```python
from build123d import *

# Parameters (mm, degrees)
SKETCH_1_W             = 43
SKETCH_1_H             = 39
BODY_DEPTH             = 1.5
SKETCH_3_R             = 1.3
OLED_PILLAR_DEPTH      = 5
OLED_WINDOW_REACH      = 31.745
SKETCH_2_W             = 34
SKETCH_2_H             = 18
SKETCH_4_W             = 43
SKETCH_4_H             = 39
SKETCH_4_W_2           = 40
SKETCH_4_H_2           = 36
FARMFEELWALL_DEPTH     = 20
MICRO5PIN_WINDOW_REACH = 53.276
SKETCH_7_W             = 12
SKETCH_7_H             = 5
RESET_WINDOW_REACH     = 50.819
SKETCH_9_W             = 6
SKETCH_9_H             = 4
SKETCH_10_W            = 15
SKETCH_10_H            = 1.5
CUT_EXTRUDE_1_DEPTH    = 2


with BuildPart() as part:
    # 스케치1 → Body (new body)
    with BuildSketch(Plane(origin=(0, 0, 0), x_dir=(1, 0, 0), z_dir=(0, 1, 0))):
        Rectangle(SKETCH_1_W, SKETCH_1_H)
    extrude(amount=BODY_DEPTH)

    # 스케치3 → OLED_pillar (add)
    with BuildSketch(Plane.XZ):
        with Locations(Location((15, 14, 0), (0, 0, 90))):
            Circle(SKETCH_3_R)
        with Locations(Location((-15, -14, 0), (0, 0, 90))):
            Circle(SKETCH_3_R)
    extrude(amount=OLED_PILLAR_DEPTH)

    # 스케치2 → OLED_window (cut, up to next)
    with BuildSketch(Plane(origin=(0, 1.5, 0), x_dir=(1, 0, 0), z_dir=(0, 1, 0)), mode=Mode.PRIVATE) as oled_window_sk1:
        with Locations((0, 1)):
            Rectangle(SKETCH_2_W, SKETCH_2_H)
    oled_window_tool1 = extrude(oled_window_sk1.sketch, amount=-OLED_WINDOW_REACH, mode=Mode.PRIVATE) & part.part
    add(oled_window_tool1.solids().sort_by_distance((0, 1.5, -1))[0], mode=Mode.SUBTRACT)

    # 스케치4 → FarmFeelWall (add)
    with BuildSketch(Plane.XZ):
        Rectangle(SKETCH_4_W, SKETCH_4_H)
        Rectangle(SKETCH_4_W_2, SKETCH_4_H_2, mode=Mode.SUBTRACT)
    extrude(amount=FARMFEELWALL_DEPTH)

    # 스케치7 → micro5pin_window (cut, up to next)
    with BuildSketch(Plane.ZY.offset(21.5), mode=Mode.PRIVATE) as micro5pin_window_sk1:
        with Locations((2.5, -8.5)):
            Rectangle(SKETCH_7_W, SKETCH_7_H)
    micro5pin_window_tool1 = extrude(micro5pin_window_sk1.sketch, amount=-MICRO5PIN_WINDOW_REACH, mode=Mode.PRIVATE) & part.part
    add(micro5pin_window_tool1.solids().sort_by_distance((-21.5, -8.5, 2.5))[0], mode=Mode.SUBTRACT)

    # 스케치9 → reset_window (cut, up to next)
    with BuildSketch(Plane.XY.offset(19.5), mode=Mode.PRIVATE) as reset_window_sk1:
        with Locations((-16, -8)):
            Rectangle(SKETCH_9_W, SKETCH_9_H)
    reset_window_tool1 = extrude(reset_window_sk1.sketch, amount=-RESET_WINDOW_REACH, mode=Mode.PRIVATE) & part.part
    add(reset_window_tool1.solids().sort_by_distance((-16, -8, 19.5))[0], mode=Mode.SUBTRACT)

    # 스케치10 → 컷-돌출1 (cut)
    with BuildSketch(Plane.XZ.offset(20)):
        with Locations((0, -18.75)):
            Rectangle(SKETCH_10_W, SKETCH_10_H)
        with Locations((0, 18.75)):
            Rectangle(SKETCH_10_W, SKETCH_10_H)
    extrude(amount=-CUT_EXTRUDE_1_DEPTH, mode=Mode.SUBTRACT)


solid = part.part
```
The listing builds one solid part. Answer for the finished solid, in the listing's coordinates (mm). A direction names the side the tool comes from. Round coordinates to 2 decimals unless told otherwise and drop trailing zeros. Loops run counter-clockwise (first coordinate to the right, second up) from the corner with the lowest first, then second, coordinate; pieces in that order, holes last.
Q1. Section C-C, the plane y = -3 is taken. Determine the outline of the cut face in (x, z).
Q2. Which of the six approach directions +Z, -Z, +X, -X, +Y, -Y give full straight-line access (tool end or side, diameter ignored) to faces 1 (the face through (-16, -10, 19)), 2 (the face through (15, -5, 14)), 3 (the face through (0, -18, -19)), 4 (the face through (0, -9, 19.5)), 5 (the face through (0, 1, -10))?
Q3. Section B-B, the plane y = -8 is taken. Determine the outline of the cut face in (x, z).
Q4. Section A-A, the plane z = -5.5 is taken. Determine the outline of the cut face in (x, y).
Q5. Find the intervals of material crossed by line 1 (Z direction, x = 5, y = -2.75); line 2 (X direction, y = -3.5, z = -3.5); line 3 (Z direction, x = 14.5, y = 0.5), in increasing order.
Q6. For a pull along Y with two mould halves and no side action, classify faces 6 (the face through (-15, -5, -14)), 7 (the face through (-21, -9, 8.5)), 8 (the face through (0, 1, 8)) as released by +Y, released by -Y, zero draft, split by the parting line, or undercut.
Q7. Given pin 1 Ø4 at (x, z) = (3, -11) entering from -Y; pin 2 Ø1.5 at (x, z) = (16, 5.5) entering from +Y; pin 3 Ø1.6 at (x, z) = (-3, -19) entering from -Y, each flat-ended and moving along its own axis, determine where each tip first touches the part or whether it passes through.
Q8. Section D-D, the plane x = -18 is taken. Determine the outline of the cut face in (y, z), then the cut area to 4 significant figures.
Completed:
1. outline: (-21.5, -19.5) - (21.5, -19.5) - (21.5, 19.5) - (-21.5, 19.5) - close; circle Ø2.6 at (-15, -14); circle Ø2.6 at (15, 14); hole (-20, -18) - (20, -18) - (20, 18) - (-20, 18) - close
2. face 1: +Z
2. face 2: -Y
2. face 3: +Z, -Z, -Y
2. face 4: +Z, +X, -X, +Y, -Y
2. face 5: +Y, -Y
3. outline: (-21.5, -19.5) - (21.5, -19.5) - (21.5, 19.5) - (-13, 19.5) - (-13, 18) - (20, 18) - (20, -18) - (-20, -18) - (-20, -3.5) - (-21.5, -3.5) - close; (-21.5, 8.5) - (-20, 8.5) - (-20, 18) - (-19, 18) - (-19, 19.5) - (-21.5, 19.5) - close
4. outline: (-21.5, -20) - (-20, -20) - (-20, 0) - (-17, 0) - (-17, 1.5) - (-21.5, 1.5) - close; (17, 0) - (20, 0) - (20, -20) - (21.5, -20) - (21.5, 1.5) - (17, 1.5) - close
5. line 1: z = -19.5 to -18, 18 to 19.5
5. line 2: x = -21.5 to -20, 20 to 21.5
5. line 3: z = -19.5 to -10, 8 to 19.5
6. face 6: released by -Y
6. face 7: undercut
6. face 8: zero draft
7. pin 1: stops at y = 0
7. pin 2: passes through
7. pin 3: stops at y = -18
8. outline: (-20, -19.5) - (1.5, -19.5) - (1.5, 19.5) - (-6, 19.5) - (-6, 18) - (0, 18) - (0, -18) - (-20, -18) - close; (-20, 18) - (-10, 18) - (-10, 19.5) - (-20, 19.5) - close
8. area: 112.5 mm2
